```python
from build123d import *

# Parameters (mm, degrees)
F0_W     = 76.2
F0_H     = 9.525
F1_DEPTH = 38.1
F2_W     = 50.8
F2_H     = 76.2
F3_DEPTH = 63.5
F4_SIZE2 = 38.1
F4_SIZE  = 38.1
F5_R     = 19.05
F6_DEPTH = 190.246
F7_SIZE  = 25.4


with BuildPart() as f1:
    # F0 (on Front) → F1 (new body, symmetric)
    with BuildSketch(Plane.XZ):
        Rectangle(F0_W, F0_H)
    extrude(amount=F1_DEPTH, both=True)

    # F2 (on face) → F3 (join)
    with BuildSketch(Plane.XY.offset(4.7625)):
        Rectangle(F2_W, F2_H)
    extrude(amount=F3_DEPTH)

    # F4
    f4_edges = [f1.edges().sort_by_distance(p)[0] for p in [
        (0, -38.1, 68.2625),
    ]]
    chamfer(f4_edges, length=F4_SIZE, length2=F4_SIZE2)

    # F5 (on face) → F6 (cut)
    with BuildSketch(Plane(origin=(0, -34.13125, 34.13125), x_dir=(1, 0, 0), z_dir=(0, -0.707107, 0.707107))):
        with Locations((0, 17.24734)):
            Circle(F5_R)
    extrude(amount=-F6_DEPTH, mode=Mode.SUBTRACT)

    # F7
    f7_edges = [f1.edges().sort_by_distance(p)[0] for p in [
        (0, 38.1, 68.2625),
    ]]
    chamfer(f7_edges, length=F7_SIZE)


solid = f1.part
```
CAD build for the part. Positions are in the model's coordinates, mm. A direction names the side the tool comes from. Round coordinates to 2 decimals unless told otherwise and drop trailing zeros. Order: outer loops, then holes, each group sorted by start corner. A loop starts at its lowest first (then second) coordinate and runs counter-clockwise, first axis right, second up. Notation, with made-up numbers: (53, 50) - (68, 50) arc R14 cw to (68, 68) - close; hole circle Ø4 at (35.5, 35). An arc over 180 degrees is marked (long way). Use CSV: the item, a comma, the result in double quotes. Start each with the question number.
1) Pin check, flat tips, straight feed: pin 1 Ø14 at (x, y) = (33.5, 8.5) entering from +Z; pin 2 Ø19 at (y, z) = (6.5, 31) entering from -X; pin 3 Ø6 at (x, z) = (2.5, 52.5) entering from -Y; pin 4 Ø1.5 at (x, z) = (-27.5, 41) entering from +Y. Stop position of each tip, or through.
2) Saw through at D-D (x = -23). List the corners of the cut face in (y, z).
3) Wall check: L1, parallel to Z at x = -33.5, y = -12.5; L2, parallel to X at y = -23.5, z = 16.5; L3, parallel to Y at x = 11, z = 15. Give the ranges that are in metal, low to high. Write a range as [from, to].
4) Saw through at A-A (x = -13.5). List the corners of the cut face in (y, z).
5) Saw through at C-C (x = 0). List the corners of the cut face in (y, z).
6) Saw through at B-B (x = 31). List the corners of the cut face in (y, z).
7) Two-plate mould, pull along Y, no slides. Class faces 1 (the flat face through (-1, 38.1, 19)), 2 (the flat face through (-1, -38.1, 13)), 3 (the cylindrical face through (10.24, 10.64, 36.47)), 4 (the flat face through (25.4, -1, 29)): pulls with the +Y half, pulls with the -Y half, needs draft (parallel to the pull), parting line crosses it, or undercut.
8) Tool access for faces 5 (the flat face through (-0.36, 25.58, 55.38)), 6 (the flat face through (-25.4, -1, 29)), 7 (the flat face through (32, -1, 4.762)): list every direction of +Z, -Z, +X, -X, +Y, -Y with a clear straight run to the whole face (end or side of a thin tool).
Values follow:
1,pin 1,"stops at z = 4.76"
1,pin 2,"stops at x = -25.4"
1,pin 3,"stops at y = -4.47"
1,pin 4,"passes through"
2,outline,"(-38.1, -4.76) - (38.1, -4.76) - (38.1, 42.86) - (12.7, 68.26) - (0, 68.26) - (-38.1, 30.16) - close"
3,L1,"z = [-4.76, 4.76]"
3,L2,"x = [-25.4, 25.4]"
3,L3,"y = [-38.1, -12.6], [31.39, 38.1]"
4,outline,"(-38.1, -4.76) - (10.15, -4.76) - (-31.44, 36.82) - (-38.1, 30.16) - close; (-12.43, 55.83) - (38.1, 5.3) - (38.1, 42.86) - (12.7, 68.26) - (0, 68.26) - close"
5,outline,"(-38.1, -4.76) - (2.21, -4.76) - (-35.41, 32.86) - (-38.1, 30.16) - close; (-8.47, 59.8) - (38.1, 13.23) - (38.1, 42.86) - (12.7, 68.26) - (0, 68.26) - close"
6,outline,"(-38.1, -4.76) - (38.1, -4.76) - (38.1, 4.76) - (-38.1, 4.76) - close"
7,face 1,"pulls with the +Y half"
7,face 2,"pulls with the -Y half"
7,face 3,"undercut"
7,face 4,"needs draft"
8,face 5,"+Z, +X, -X, +Y"
8,face 6,"+Z, -X, +Y, -Y"
8,face 7,"+Z, +X, +Y, -Y"
